Autodesk Inventor part; units mm, degrees
ref_plane "YZ Plane" through (0, 0, 0) normal (1, 0, 0) x (0, 1, 0)
ref_plane "XZ Plane" through (0, 0, 0) normal (0, 1, 0) x (-1, 0, 0)
ref_plane "XY Plane" through (0, 0, 0) normal (0, 0, 1) x (1, 0, 0)
sketch "Sketch1" plane through (0, 0, 0) normal (0, 0, 1) x (1, 0, 0)
  line L0 (0, 0) -> (25.4, 0)
  line L1 (25.4, 0) -> (25.4, 457.2)
  line L2 (25.4, 457.2) -> (0, 457.2)
  line L3 (0, 457.2) -> (0, 0)
  dimension "d0" = 457.2
  dimension "d1" = 25.4
extrude "Extrusion1" add sketch "Sketch1" along normal blind 25.4
shell "Shell1" thickness 1.5875 removed faces 2 at (16.9333, 457.2, 8.4667) at (8.4667, 0, 8.4667)
properties part number "Frame_VerticalSideGuide_Long" material "Aluminum-6061"
Verification items for the finished model (mm, model axes). A direction names the side the tool comes from. Coordinates: 2 decimals unless noted, no trailing zeros. Loops run counter-clockwise (first coordinate to the right, second up) from the corner with the lowest first, then second, coordinate; pieces in that order, holes last. Notation, with made-up numbers: (-30, 61) - (-7, 61) arc R34 ccw to (-7, 95) - close; hole circle Ø10 at (-39.5, 12). An arc over 180 degrees is marked (long way). Put each result on its own line as item: value.
Item 1: Section check C-C (z = 18.25). Enter the section's corners in (x, y), then the cut area to 3 significant figures.
Conclusion:
outline: (0, 0) - (1.59, 0) - (1.59, 457.2) - (0, 457.2) - close; (23.81, 0) - (25.4, 0) - (25.4, 457.2) - (23.81, 457.2) - close
area: 1,450 mm2
Item 2: Section check A-A (x = 18.5). Enter the section's corners in (y, z), then the cut area to 3 significant figures.
Conclusion:
outline: (0, 0) - (457.2, 0) - (457.2, 1.59) - (0, 1.59) - close; (0, 23.81) - (457.2, 23.81) - (457.2, 25.4) - (0, 25.4) - close
area: 1,450 mm2
Item 3: Section check B-B (y = 130.5). Enter the section's corners in (x, z).
Conclusion:
outline: (0, 0) - (25.4, 0) - (25.4, 25.4) - (0, 25.4) - close; hole (1.59, 1.59) - (23.81, 1.59) - (23.81, 23.81) - (1.59, 23.81) - close
Item 4: Set-up check for faces 1 (the face through (1, 0, 13)), 2 (the face through (13, 232, 1.588)): record each of +Z, -Z, +X, -X, +Y, -Y from which the full face is reachable in a straight line by a thin tool's end or side.
Conclusion:
face 1: +Z, -Z, +X, -X, -Y
face 2: +Y, -Y
Item 5: Scan line: line 1 along X through (y, z) = (295.5, 12.5). Record every from-to range of solid material in increasing order.
Conclusion:
line 1: x = 0 to 1.59, 23.81 to 25.4
Item 6: Draft check along Z on faces 3 (the face through (23.812, 225, 13)), 4 (the face through (24, 457.2, 13)), 5 (the face through (13, 232, 0)). Enter one of: pulls with the +Z half, pulls with the -Z half, needs draft (parallel to the pull), parting line crosses it, or undercut.
Conclusion:
face 3: undercut
face 4: needs draft
face 5: pulls with the -Z half
